Part model, mm, in its own coordinate system. Face numbers are marked on the shaded views. A direction names the side the tool comes from. Give positions to 0.01 mm unless a question says otherwise; leave off trailing zeros. Order: outer loops, then holes, each group sorted by start corner. A loop starts at its lowest first (then second) coordinate and runs counter-clockwise, first axis right, second up. Notation, with made-up numbers: M 68.25,68.25 L 103.25,68.25 A13 ccw 103.25,91.25 Z; hole C 16.25,46 d7. An arc over 180 degrees is marked long. Answer as a JSON object with one key per item and string values.
from build123d import *

# Parameters (mm, degrees)
BOSS_EXTRUDE1_DEPTH = 65
BOSS_EXTRUDE2_DEPTH = 65
SKETCH3_W           = 62.5
SKETCH3_H           = 30
CUT_EXTRUDE1_DEPTH  = 65
SKETCH5_W           = 80
SKETCH5_H           = 120
CUT_EXTRUDE2_DEPTH  = 60
SKETCH6_R           = 6
CUT_EXTRUDE3_DEPTH  = 25
FILLET1_R           = 33
SKETCH7_R           = 15
CUT_EXTRUDE4_DEPTH  = 10
SKETCH8_R           = 23.75
CUT_EXTRUDE5_DEPTH  = 10
SKETCH10_W          = 22.5
SKETCH10_H          = 55
CUT_EXTRUDE7_DEPTH  = 25
SKETCH11_R          = 20
CUT_EXTRUDE8_DEPTH  = 5
SKETCH12_R          = 30
BOSS_EXTRUDE3_DEPTH = 5
SKETCH13_R          = 22.5
BOSS_EXTRUDE4_DEPTH = 15
SKETCH14_W          = 10
SKETCH14_H          = 20
BOSS_EXTRUDE5_DEPTH = 65
SKETCH15_R          = 5
CUT_EXTRUDE9_DEPTH  = 10


with BuildPart() as part:
    # Sketch1 → Boss-Extrude1 (new body)
    with BuildSketch(Plane.XY):
        Polygon((-59.142135624, 0), (59.142135624, 0), (81.25, -22.107864376), (81.25, -201.25), (71.25, -201.25), (71.25, -26.25), (55, -10), (-55, -10), (-71.25, -26.25), (-71.25, -201.25), (-81.25, -201.25), (-81.25, -22.107864376), align=None)
    extrude(amount=BOSS_EXTRUDE1_DEPTH)

    # Sketch2 → Boss-Extrude2 (add)
    with BuildSketch(Plane.XY):
        Polygon((68.75, -9.607864376), (68.75, 165.392135624), (8.75, 165.392135624), (8.75, 177.892135624), (-16.25, 177.892135624), (-16.25, 0), (59.142135624, 0), align=None)
    extrude(amount=BOSS_EXTRUDE2_DEPTH)

    # Sketch3 → Cut-Extrude1 (cut)
    with BuildSketch(Plane.XY.offset(65)):
        with Locations((27.5, 15)):
            Rectangle(SKETCH3_W, SKETCH3_H)
    extrude(amount=-CUT_EXTRUDE1_DEPTH, mode=Mode.SUBTRACT)

    # Sketch5 → Cut-Extrude2 (cut)
    with BuildSketch(Plane.XY.offset(65)):
        with Locations((23.75, 97.892135624)):
            Rectangle(SKETCH5_W, SKETCH5_H)
    extrude(amount=-CUT_EXTRUDE2_DEPTH, mode=Mode.SUBTRACT)

    # Sketch6 → Cut-Extrude3 (cut)
    with BuildSketch(Plane.ZY.offset(16.25)):
        with Locations(Location((30, 164.892135624, 0), (0, 0, 270))):
            Circle(SKETCH6_R)
        with Locations(Location((30, 29.942135624, 0), (0, 0, 179.447427343))):
            Circle(SKETCH6_R)
    extrude(amount=-CUT_EXTRUDE3_DEPTH, mode=Mode.SUBTRACT)

    # Fillet1
    # the kernel refuses this fillet: 33 mm, written as the material it takes off along each edge
    with BuildSketch(Plane(origin=(163.75, -201.25, 65), x_dir=(0, 1, 0), z_dir=(-1, 0, 0)), Plane(origin=(11.25, -201.25, 65), x_dir=(0, 1, 0), z_dir=(-1, 0, 0))) as fillet1_piece_1:
        with BuildLine():
            CenterArc((FILLET1_R, FILLET1_R), FILLET1_R, 180, 90)
            Line((0, FILLET1_R), (0, 0))
            Line((0, 0), (FILLET1_R, 0))
        make_face()
    extrude(amount=175, mode=Mode.SUBTRACT)
    with BuildSketch(Plane(origin=(163.75, -201.25, 0), x_dir=(0, 1, 0), z_dir=(-1, 0, 0)), Plane(origin=(11.25, -201.25, 0), x_dir=(0, 1, 0), z_dir=(-1, 0, 0))) as fillet1_piece_2:
        with BuildLine():
            CenterArc((FILLET1_R, -FILLET1_R), FILLET1_R, 90, 90)
            Line((0, -FILLET1_R), (0, 0))
            Line((0, 0), (FILLET1_R, 0))
        make_face()
    extrude(amount=175, mode=Mode.SUBTRACT)

    # Sketch7 → Cut-Extrude4 (cut)
    with BuildSketch(Plane.ZY.offset(81.25)):
        with Locations((33, -168.25)):
            Circle(SKETCH7_R)
    extrude(amount=-CUT_EXTRUDE4_DEPTH, mode=Mode.SUBTRACT)

    # Sketch8 → Cut-Extrude5 (cut)
    with BuildSketch(Plane(origin=(81.25, 0, 0), x_dir=(0, 0, -1), z_dir=(1, 0, 0))):
        with Locations((-32, -168.25)):
            Circle(SKETCH8_R)
    extrude(amount=-CUT_EXTRUDE5_DEPTH, mode=Mode.SUBTRACT)

    # Sketch10 → Cut-Extrude7 (cut)
    with BuildSketch(Plane(origin=(0, 165.392135624, 0), x_dir=(1, 0, 0), z_dir=(0, 1, 0))):
        with Locations((50, -37.5)):
            Rectangle(SKETCH10_W, SKETCH10_H)
    extrude(amount=-CUT_EXTRUDE7_DEPTH, mode=Mode.SUBTRACT)

    # Sketch11 → Cut-Extrude8 (cut)
    with BuildSketch(Plane(origin=(68.75, 0, 0), x_dir=(0, 0, -1), z_dir=(1, 0, 0))):
        with Locations((-32.5, 65.392135624)):
            Circle(SKETCH11_R)
    extrude(amount=-CUT_EXTRUDE8_DEPTH, mode=Mode.SUBTRACT)

    # Sketch12 → Boss-Extrude3 (add)
    with BuildSketch(Plane(origin=(68.75, 0, 0), x_dir=(0, 0, -1), z_dir=(1, 0, 0))):
        with Locations(Location((-32.5, 118.286013704, 0), (0, 0, 180))):
            Circle(SKETCH12_R)
    extrude(amount=BOSS_EXTRUDE3_DEPTH)

    # Sketch13 → Boss-Extrude4 (add)
    with BuildSketch(Plane(origin=(73.75, 0, 0), x_dir=(0, 0, -1), z_dir=(1, 0, 0))):
        with Locations((-32.5, 118.286013704)):
            Circle(SKETCH13_R)
    extrude(amount=BOSS_EXTRUDE4_DEPTH)

    # Sketch14 → Boss-Extrude5 (add)
    with BuildSketch(Plane.XY):
        with Locations((66.25, -85)):
            Rectangle(SKETCH14_W, SKETCH14_H)
    extrude(amount=BOSS_EXTRUDE5_DEPTH)

    # Sketch15 → Cut-Extrude9 (cut)
    with BuildSketch(Plane(origin=(81.25, 0, 0), x_dir=(0, 0, -1), z_dir=(1, 0, 0))):
        with Locations((-32.5, -113.83)):
            Circle(SKETCH15_R)
    extrude(amount=-CUT_EXTRUDE9_DEPTH, mode=Mode.SUBTRACT)


solid = part.part
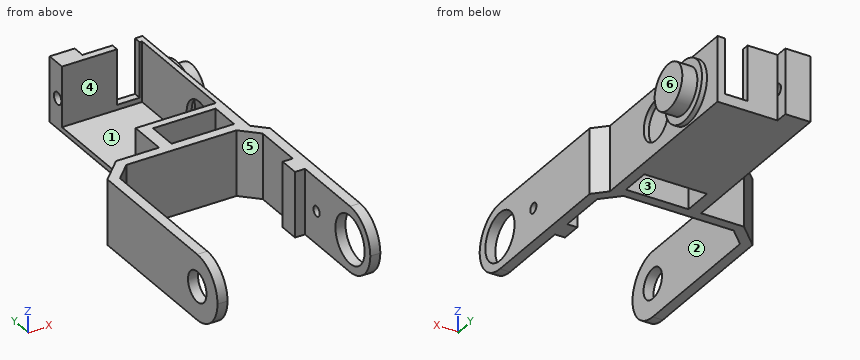
1. Which spindle directions (+Z, -Z, +X, -X, +Y, -Y) get a long thin tool onto all of the face, cutting with end or side? Do the marked faces 1, 2 and 3. Say none if no direction does.
Worked answers:
{"face 1": "+Z, -X", "face 2": "+Z, -Z, -Y", "face 3": "+Z, -Z"}
2. Probe line 1 along Y through (x, z) = (24, 25); line 2 along Y through (x, z) = (1.75, 30); line 3 along Y through (x, z) = (-9.25, 30). List the from-to ranges inside material, lowest first.
Worked answers:
{"line 1": "y = -10 to 0, 30 to 37.89, 157.89 to 165.39", "line 2": "y = -10 to 0, 35.94 to 37.89, 157.89 to 158.89, 170.89 to 177.89", "line 3": "y = -10 to 23.94, 35.94 to 37.89, 157.89 to 158.89, 170.89 to 177.89"}
3. Cut at A-A on x = 21.5. Give the cut face in (y, z), plus the area to 3 significant figures.
Worked answers:
{"outline": "M -10,0 L 0,0 L 0,65 L -10,65 Z; M 30,0 L 165.39,0 L 165.39,65 L 157.89,65 L 157.89,5 L 37.89,5 L 37.89,65 L 30,65 Z", "area": "2,250 mm^2"}
4. Pin check, flat tips, straight feed: P1, Ø10, axis at y = -41.5, z = 23.5, coming from the +X side; P2, Ø5, axis at x = 68, z = 18, coming from the -Y side; P3, Ø4, axis at x = 2, z = 11, coming from the -Y side. Stop position of each tip, or through.
Worked answers:
{"P1": "stops at x = 81.25", "P2": "stops at y = -95", "P3": "stops at y = -10"}
5. Two-plate mould, pull along X, no slides. Class the marked faces 4, 5 and 6: +X half, -X half, draft (parallel to the pull), parting line (faces both ways), or undercut.
Worked answers:
{"face 4": "draft", "face 5": "undercut", "face 6": "+X half"}
6. Cut at C-C on y = 79.5. Give the cut face in (x, z).
Worked answers:
{"outline": "M -16.25,0 L 68.75,0 L 68.75,18.32 L 63.75,18.32 L 63.75,5 L -16.25,5 Z; M 63.75,46.68 L 68.75,46.68 L 68.75,65 L 63.75,65 Z"}
7. Cut at B-B on y = -113.83. Give the cut face in (x, z).
Worked answers:
{"outline": "M -81.25,0 L -71.25,0 L -71.25,65 L -81.25,65 Z; M 71.25,0 L 81.25,0 L 81.25,27.5 L 71.25,27.5 Z; M 71.25,37.5 L 81.25,37.5 L 81.25,65 L 71.25,65 Z"}
8. Cut at D-D on y = -174.5. Give the cut face in (x, z), plus the area to 3 significant figures.
Worked answers:
{"outline": "M -81.25,0.6 L -71.25,0.6 L -71.25,19.36 L -81.25,19.36 Z; M -81.25,46.64 L -71.25,46.64 L -71.25,64.4 L -81.25,64.4 Z; M 71.25,0.6 L 81.25,0.6 L 81.25,9.09 L 71.25,9.09 Z; M 71.25,54.91 L 81.25,54.91 L 81.25,64.4 L 71.25,64.4 Z", "area": "545 mm^2"}
